from build123d import *

# Parameters (mm, degrees)
SKETCH_1_R           = 3.5
EXTRUDE_1_DEPTH      = 39
SKETCH_2_R           = 1.5
EXTRUDE_3_DEPTH      = 4
EXTRUDE_3_DEPTH_BACK = 43


with BuildPart() as part:
    # 草图1 → 凸台-拉伸1 (new body)
    with BuildSketch(Plane.XY):
        Circle(SKETCH_1_R)
    extrude(amount=EXTRUDE_1_DEPTH)

    # 草图2 → 凸台-拉伸3 (add, two sides)
    with BuildSketch(Plane.XY.offset(39)) as extrude_3_sk:
        Circle(SKETCH_2_R)
    extrude(amount=EXTRUDE_3_DEPTH)
    extrude(extrude_3_sk.sketch, amount=-EXTRUDE_3_DEPTH_BACK)


solid = part.part
The model under review builds one solid part; all positions refer to its coordinate system, in mm. A direction names the side the tool comes from. Round coordinates to 2 decimals unless told otherwise and drop trailing zeros. Loops run counter-clockwise (first coordinate to the right, second up) from the corner with the lowest first, then second, coordinate; pieces in that order, holes last. Notation, with made-up numbers: M -34,78 L 2,78 A24 ccw 2,88 Z; hole C 70.25,-38 d4. An arc over 180 degrees is marked long. Answer as a JSON object with one key per item and string values.
Item 1: We need section C-C, the plane z = 24. State the section outline as (x, y) points.
Check sheet entries:
{"outline": "C 0,0 d7"}
Item 2: Tool access review of faces 1 (the face through (0, -2, 0)), 2 (the face through (0, 0, -4)), 3 (the face through (0, -2, 39)): name each direction out of +Z, -Z, +X, -X, +Y, -Y from which nothing blocks a thin tool from reaching the whole face with its end or side.
Check sheet entries:
{"face 1": "-Z", "face 2": "-Z, +X, -X, +Y, -Y", "face 3": "+Z"}
Item 3: We need section D-D, the plane y = -2.5. State the section outline as (x, z) points, and give its area (3 significant figures).
Check sheet entries:
{"outline": "M -2.45,0 L 2.45,0 L 2.45,39 L -2.45,39 Z", "area": "191 mm2"}
Item 4: For line 1 along Z through (x, y) = (1.5, 2.5); line 2 along Y through (x, z) = (-0.25, 15.5), list the stretches that pass through material, from the lowest coordinate up.
Check sheet entries:
{"line 1": "0 to 39", "line 2": "-3.49 to 3.49"}
Item 5: We need section A-A, the plane y = 0. State the section outline as (x, z) points.
Check sheet entries:
{"outline": "M -3.5,0 L -1.5,0 L -1.5,-4 L 1.5,-4 L 1.5,0 L 3.5,0 L 3.5,39 L 1.5,39 L 1.5,43 L -1.5,43 L -1.5,39 L -3.5,39 Z"}
Item 6: Clearance check with flat-ended pins moving along their axes: P1, Ø1, axis at y = -2, z = 21, coming from the -X side; P2, Ø1, axis at x = 3, z = 15.5, coming from the +Y side. State where each tip first meets the part, or that it passes through.
Check sheet entries:
{"P1": "x = -3.16", "P2": "y = 2.45"}
